from build123d import *

# Parameters (mm, degrees)
SKETCH1_W           = 39
SKETCH1_H           = 30
SKETCH1_R           = 10.45
BOSS_EXTRUDE1_DEPTH = 6.4
BOSS_EXTRUDE2_DEPTH = 14.6
CUT_EXTRUDE1_DEPTH  = 6.4
FILLET1_R           = 2
FILLET2_R           = 1


with BuildPart() as part:
    # Sketch1 → Boss-Extrude1 (new body)
    with BuildSketch(Plane(origin=(0, 0, 0), x_dir=(1, 0, 0), z_dir=(0, 1, 0))):
        Rectangle(SKETCH1_W, SKETCH1_H)
        with Locations(Location((0, 0, 0), (0, 0, 270))):
            Circle(SKETCH1_R, mode=Mode.SUBTRACT)
    extrude(amount=BOSS_EXTRUDE1_DEPTH)

    # Sketch2 → Boss-Extrude2 (add)
    with BuildSketch(Plane.XY.offset(15)):
        Polygon((-13, 0), (-14.5, -9), (-14.5, -24), (14.5, -24), (14.5, -9), (13, 0), align=None)
    extrude(amount=-BOSS_EXTRUDE2_DEPTH)

    # Sketch3 → Cut-Extrude1 (cut)
    with BuildSketch(Plane(origin=(0, 6.4, 0), x_dir=(1, 0, 0), z_dir=(0, 1, 0))):
        with BuildLine():
            Line((19.5, 5.45), (19.5, -5.45))
            ThreePointArc((19.5, -5.45), (16.892891986, 0), (19.5, 5.45))
        make_face()
    extrude(amount=-CUT_EXTRUDE1_DEPTH, mode=Mode.SUBTRACT)

    # Fillet1
    fillet1_edges = [part.edges().sort_by_distance(p)[0] for p in [
        (19.5, 3.2, -5.45),
        (19.5, 3.2, 5.45),
        (19.5, 3.2, 15),
        (-19.5, 3.2, 15),
        (-19.5, 3.2, -15),
        (19.5, 3.2, -15),
    ]]
    fillet(fillet1_edges, radius=FILLET1_R)

    # Fillet2
    fillet2_edges = [part.edges().sort_by_distance(p)[0] for p in [
        (14.5, -9, 7.7),
        (14.5, -24, 7.7),
        (-14.5, -24, 7.7),
        (-14.5, -9, 7.7),
    ]]
    fillet(fillet2_edges, radius=FILLET2_R)


solid = part.part
Part model, mm, in its own coordinate system. A direction names the side the tool comes from. Coordinates: 2 decimals unless noted, no trailing zeros. Order: outer loops, then holes, each group sorted by start corner. A loop starts at its lowest first (then second) coordinate and runs counter-clockwise, first axis right, second up. Notation, with made-up numbers: M 87.5,62.25 L 123.5,62.25 A24 ccw 123.5,80.25 Z; hole C 43.5,71 d8. An arc over 180 degrees is marked long. One line per question, with ' | ' between items.
Q1. 3-axis set-ups, long thin cutter, end or side, ignore diameter. For faces 4 (the face through (-13.733, -4.397, 7.802)), 5 (the face through (0, -12, 0.4)), 6 (the face through (0, 0, 4)), 7 (the face through (19.345, 3.155, 5.564)): which of +Z, -Z, +X, -X, +Y, -Y reach the whole face in a straight line?
A:
face 4: +Z, -Z, -X | face 5: -Z, +X, -X, -Y | face 6: +Y | face 7: +X, +Y, -Y
Q2. Slice it at C-C (z = -3). Give the cut face in (x, y), and give its area (3 significant figures).
A:
outline: M -19.5,0 L -10.01,0 L -10.01,6.4 L -19.5,6.4 Z; M 10.01,0 L 17.57,0 L 17.57,6.4 L 10.01,6.4 Z | area: 109 mm^2
Q3. Pin check, flat tips, straight feed: P1, Ø8, axis at y = -11.5, z = 11.5, coming from the +X side; P2, Ø1.5, axis at y = -3.5, z = -0.5, coming from the -X side; P3, Ø10, axis at x = -12.5, y = -9, coming from the -Z side; P4, Ø5, axis at x = 3.5, z = 4.5, coming from the +Y side. Stop position of each tip, or through.
A:
P1: stops at x = 14.5 | P2: passes through | P3: stops at z = 0.4 | P4: stops at y = 0
Q4. Slice it at A-A (x = 0). Give the cut face in (y, z), and give its area (3 significant figures).
A:
outline: M -24,0.4 L 0,0.4 L 0,10.45 L 6.4,10.45 L 6.4,15 L -24,15 Z; M 0,-15 L 6.4,-15 L 6.4,-10.45 L 0,-10.45 Z | area: 409 mm^2
Q5. Drill centre lines: line 1 (X direction, y = 2.5, z = 0); line 2 (Y direction, x = 16, z = 13); line 3 (Z direction, x = -1, y = 5). Where is each one in solid material? Low to high.
A:
line 1: x = -19.5 to -10.45, 10.45 to 16.89 | line 2: y = 0 to 6.4 | line 3: z = -15 to -10.4, 10.4 to 15
Q6. Slice it at B-B (y = 1.5). Give the cut face in (x, z).
A:
outline: M -19.5,-13 A2 ccw -17.5,-15 L 17.5,-15 A2 ccw 19.5,-13 L 19.5,-6.33 A2 ccw 18.92,-4.93 A7 cw 18.92,4.93 A2 ccw 19.5,6.33 L 19.5,13 A2 ccw 17.5,15 L -17.5,15 A2 ccw -19.5,13 Z; hole C 0,0 d20.9
Q7. Two-plate mould, pull along X, no slides. Class faces 1 (the face through (-5, 0, -10)), 2 (the face through (3.139, 3.155, 9.967)), 3 (the face through (-14.5, -16, 8)): +X half, -X half, draft (parallel to the pull), parting line (faces both ways), or undercut.
A:
face 1: draft | face 2: undercut | face 3: -X half
Q8. Slice it at D-D (x = 9.5). Give the cut face in (y, z), and give its area (3 significant figures).
A:
outline: M -24,0.4 L 0,0.4 L 0,4.35 L 6.4,4.35 L 6.4,15 L -24,15 Z; M 0,-15 L 6.4,-15 L 6.4,-4.35 L 0,-4.35 Z | area: 487 mm^2
